Geometry: final body of the model. Coordinates: model frame, mm. A direction names the side the tool comes from. Give positions to 0.01 mm unless a question says otherwise; leave off trailing zeros. Order: outer loops, then holes, each group sorted by start corner. A loop starts at its lowest first (then second) coordinate and runs counter-clockwise, first axis right, second up. Notation, with made-up numbers: M 39,16.25 L 94,16.25 A20 cw 94,43.25 Z; hole C 70.25,-12.5 d4. An arc over 180 degrees is marked long. Write item = value, one per line. Start each with the question number.
from build123d import *

# Parameters (mm, degrees)
SKETCH_1_W            = 28
SKETCH_1_H            = 46
SKETCH_1_R            = 0.75
SKETCH_1_W_2          = 35.5
SKETCH_1_H_2          = 84
SKETCH_1_W_3          = 7
SKETCH_1_H_3          = 52
SKETCH_1_W_4          = 73
SKETCH_1_H_4          = 54
SKETCH_1_R_2          = 1
SKETCH_1_W_5          = 5
SKETCH_1_H_5          = 50
EXTRUDE_1_DEPTH       = 1
EXTRUDE_2_OUTLINE_W   = 73
EXTRUDE_2_OUTLINE_H   = 86
EXTRUDE_2_OUTLINE_W_2 = 71
EXTRUDE_2_OUTLINE_H_2 = 84
EXTRUDE_2_OUTLINE_W_3 = 1
EXTRUDE_2_OUTLINE_H_3 = 46
EXTRUDE_2_DEPTH       = 10
SKETCH_1_4_W          = 7
SKETCH_1_4_H          = 52
SKETCH_1_4_W_2        = 5
SKETCH_1_4_H_2        = 50
EXTRUDE_3_DEPTH       = 4
SKETCH_1_5_R          = 0.75
SKETCH_1_5_R_2        = 1
EXTRUDE_4_DEPTH       = 5
SKETCH_2_W            = 10
SKETCH_2_H            = 5
CUT_EXTRUDE_2_DEPTH   = 10


# Read off the part's stored shape, not the designer's step: the extrude step
with BuildPart() as part:
    # Sketch 1 → Extrude 1 (new body)
    # profile 1 of 10: a face of its own
    with BuildSketch(Plane(origin=(0, 0, 0), x_dir=(1, 0, 0), z_dir=(0, 1, 0))):
        with Locations((-15, 62)):
            Rectangle(SKETCH_1_W, SKETCH_1_H)
        with Locations(Location((-24, 43, 0), (0, 0, 270))):
            Circle(SKETCH_1_R, mode=Mode.SUBTRACT)
        with Locations(Location((-4, 43, 0), (0, 0, 270))):
            Circle(SKETCH_1_R, mode=Mode.SUBTRACT)
        with Locations(Location((-24, 81, 0), (0, 0, 270))):
            Circle(SKETCH_1_R, mode=Mode.SUBTRACT)
        with Locations(Location((-4, 81, 0), (0, 0, 270))):
            Circle(SKETCH_1_R, mode=Mode.SUBTRACT)
    # profile 2 of 10: a face of its own
    with BuildSketch(Plane(origin=(0, 0, 0), x_dir=(1, 0, 0), z_dir=(0, 1, 0))):
        with Locations((17.75, 42)):
            Rectangle(SKETCH_1_W_2, SKETCH_1_H_2)
        with Locations((5.5, 28.4)):
            Rectangle(SKETCH_1_W_3, SKETCH_1_H_3, mode=Mode.SUBTRACT)
    # profile 3 of 10: a face of its own
    with BuildSketch(Plane(origin=(0, 0, 0), x_dir=(1, 0, 0), z_dir=(0, 1, 0))):
        with Locations((53.25, 42)):
            Rectangle(SKETCH_1_W_2, SKETCH_1_H_2)
        with Locations((65.5, 28.4)):
            Rectangle(SKETCH_1_W_3, SKETCH_1_H_3, mode=Mode.SUBTRACT)
    # profile 4 of 10: a face of its own
    with BuildSketch(Plane(origin=(0, 0, 0), x_dir=(1, 0, 0), z_dir=(0, 1, 0))):
        with Locations((35.5, -28)):
            Rectangle(SKETCH_1_W_4, SKETCH_1_H_4)
        with Locations(Location((6.5, -43, 0), (0, 0, 270))):
            Circle(SKETCH_1_R_2, mode=Mode.SUBTRACT)
        with Locations(Location((64.5, -43, 0), (0, 0, 270))):
            Circle(SKETCH_1_R_2, mode=Mode.SUBTRACT)
        with Locations(Location((64.5, -16, 0), (0, 0, 270))):
            Circle(SKETCH_1_R_2, mode=Mode.SUBTRACT)
        with Locations(Location((6.5, -16, 0), (0, 0, 270))):
            Circle(SKETCH_1_R_2, mode=Mode.SUBTRACT)
    # profile 5 of 10: a face of its own
    with BuildSketch(Plane(origin=(0, 0, 0), x_dir=(1, 0, 0), z_dir=(0, 1, 0))):
        Polygon((72, 85), (35.5, 85), (35.5, 84), (71, 84), (71, 0), (35.5, 0), (35.5, -1), (72, -1), align=None)
    # profile 6 of 10: a face of its own
    with BuildSketch(Plane(origin=(0, 0, 0), x_dir=(1, 0, 0), z_dir=(0, 1, 0))):
        Polygon((35.5, 85), (-1, 85), (-1, 39), (-1, -1), (35.5, -1), (35.5, 0), (0, 0), (0, 84), (35.5, 84), align=None)
    # profile 7 of 10: a face of its own
    with BuildSketch(Plane(origin=(0, 0, 0), x_dir=(1, 0, 0), z_dir=(0, 1, 0))):
        with Locations((5.5, 28.4)):
            Rectangle(SKETCH_1_W_3, SKETCH_1_H_3)
        with Locations((5.5, 28.4)):
            Rectangle(SKETCH_1_W_5, SKETCH_1_H_5, mode=Mode.SUBTRACT)
    # profile 8 of 10: a face of its own
    with BuildSketch(Plane(origin=(0, 0, 0), x_dir=(1, 0, 0), z_dir=(0, 1, 0))):
        with Locations((5.5, 28.4)):
            Rectangle(SKETCH_1_W_5, SKETCH_1_H_5)
    # profile 9 of 10: a face of its own
    with BuildSketch(Plane(origin=(0, 0, 0), x_dir=(1, 0, 0), z_dir=(0, 1, 0))):
        with Locations((65.5, 28.4)):
            Rectangle(SKETCH_1_W_3, SKETCH_1_H_3)
        with Locations((65.5, 28.4)):
            Rectangle(SKETCH_1_W_5, SKETCH_1_H_5, mode=Mode.SUBTRACT)
    # profile 10 of 10: a face of its own
    with BuildSketch(Plane(origin=(0, 0, 0), x_dir=(1, 0, 0), z_dir=(0, 1, 0))):
        with Locations((65.5, 28.4)):
            Rectangle(SKETCH_1_W_5, SKETCH_1_H_5)
    extrude(amount=EXTRUDE_1_DEPTH)

    # Extrude 2 outline → Extrude 2 (add)
    # profile 1 of 2: a face of its own
    with BuildSketch(Plane(origin=(0, 0, 0), x_dir=(1, 0, 0), z_dir=(0, 1, 0))):
        with Locations((35.5, 42)):
            Rectangle(EXTRUDE_2_OUTLINE_W, EXTRUDE_2_OUTLINE_H)
        with Locations((35.5, 42)):
            Rectangle(EXTRUDE_2_OUTLINE_W_2, EXTRUDE_2_OUTLINE_H_2, mode=Mode.SUBTRACT)
    # profile 2 of 2: a face of its own
    with BuildSketch(Plane(origin=(0, 0, 0), x_dir=(1, 0, 0), z_dir=(0, 1, 0))):
        with Locations((-29.5, 62)):
            Rectangle(EXTRUDE_2_OUTLINE_W_3, EXTRUDE_2_OUTLINE_H_3)
    extrude(amount=EXTRUDE_2_DEPTH)

    # Sketch 1_4 → Extrude 3 (add)
    # profile 1 of 2: a face of its own
    with BuildSketch(Plane(origin=(0, 0, 0), x_dir=(1, 0, 0), z_dir=(0, 1, 0))):
        with Locations((5.5, 28.4)):
            Rectangle(SKETCH_1_4_W, SKETCH_1_4_H)
        with Locations((5.5, 28.4)):
            Rectangle(SKETCH_1_4_W_2, SKETCH_1_4_H_2, mode=Mode.SUBTRACT)
    # profile 2 of 2: a face of its own
    with BuildSketch(Plane(origin=(0, 0, 0), x_dir=(1, 0, 0), z_dir=(0, 1, 0))):
        with Locations((65.5, 28.4)):
            Rectangle(SKETCH_1_4_W, SKETCH_1_4_H)
        with Locations((65.5, 28.4)):
            Rectangle(SKETCH_1_4_W_2, SKETCH_1_4_H_2, mode=Mode.SUBTRACT)
    extrude(amount=EXTRUDE_3_DEPTH)

    # Sketch 1_5 → Extrude 4 (add)
    with BuildSketch(Plane(origin=(0, 0, 0), x_dir=(1, 0, 0), z_dir=(0, 1, 0))):
        with Locations(Location((-4, 43, 0), (0, 0, 270))):
            Circle(SKETCH_1_5_R)
        with Locations(Location((-24, 43, 0), (0, 0, 270))):
            Circle(SKETCH_1_5_R)
        with Locations(Location((-24, 81, 0), (0, 0, 270))):
            Circle(SKETCH_1_5_R)
        with Locations(Location((-4, 81, 0), (0, 0, 270))):
            Circle(SKETCH_1_5_R)
        with Locations(Location((6.5, -16, 0), (0, 0, 270))):
            Circle(SKETCH_1_5_R_2)
        with Locations(Location((64.5, -16, 0), (0, 0, 270))):
            Circle(SKETCH_1_5_R_2)
        with Locations(Location((64.5, -43, 0), (0, 0, 270))):
            Circle(SKETCH_1_5_R_2)
        with Locations(Location((6.5, -43, 0), (0, 0, 270))):
            Circle(SKETCH_1_5_R_2)
    extrude(amount=EXTRUDE_4_DEPTH)

    # Sketch 2 → Cut-Extrude 2 (cut)
    with BuildSketch(Plane.XY.offset(-84)):
        with Locations((48, 7.5)):
            Rectangle(SKETCH_2_W, SKETCH_2_H)
    extrude(amount=-CUT_EXTRUDE_2_DEPTH, mode=Mode.SUBTRACT)


solid = part.part
1) Draft query along X for faces 4 (the flat face through (35, 5, 1)), 5 (the flat face through (69, 2, -28)). Return one class per face: pulls with the +X half, pulls with the -X half, needs draft (parallel to the pull), parting line crosses it, or undercut.
2) Cut plane C-C (z = 3). Return loops of the section in (x, y).
3) Cut plane A-A (z = -75). Return loops of the section in (x, y), plus the area to 3 significant figures.
4) Cut plane B-B (x = 36). Return loops of the section in (y, z), plus the area to 3 significant figures.
5) Cut plane D-D (x = -21.5). Return loops of the section in (y, z).
6) Access query for faces 1 (the flat face through (-19.9, 0.5, -39)), 2 (the flat face through (2, 2, -28)), 3 (the flat face through (-29, 5, -62)). Directions: +Z, -Z, +X, -X, +Y, -Y. A direction counts if a zero-diameter tool reaches every point of the face in a straight line with its end or side. Return the directions, or none.
7) Ray query, L1, parallel to X at y = 4.75, z = -42; L2, parallel to X at y = 3.25, z = -38; L3, parallel to Z at x = 9, y = 5.75. Return the intervals inside material, ascending.
8) Pin query (flat end, axial travel): pin 1 Ø5 at (y, z) = (6.5, -25) entering from -X; pin 2 Ø1.5 at (x, y) = (8.5, 6) entering from +Z; pin 3 Ø1.5 at (x, y) = (5, 2) entering from +Z. Return the tip coordinate at first contact, or that it passes through.
Reply:
q1.face_4 = needs draft
q1.face_5 = undercut
q2.outline = M -1,0 L 72,0 L 72,1 L -1,1 Z
q3.outline = M -30,0 L 72,0 L 72,10 L 71,10 L 71,1 L 0,1 L 0,10 L -1,10 L -1,1 L -29,1 L -29,10 L -30,10 Z
q3.area = 129 mm²
q4.outline = M 0,-85 L 10,-85 L 10,-84 L 1,-84 L 1,0 L 10,0 L 10,1 L 1,1 L 1,55 L 0,55 Z
q4.area = 158 mm²
q5.outline = M 0,-85 L 1,-85 L 1,-39 L 0,-39 Z
q6.face_1 = +Z, -X, +Y, -Y
q6.face_2 = +Y
q6.face_3 = +Z, -Z, +Y
q7.L1 = -30 to -29, -1 to 0, 71 to 72
q7.L2 = -1 to 0, 2 to 3, 8 to 9, 62 to 63, 68 to 69, 71 to 72
q7.L3 = -85 to -84, 0 to 1
q8.pin_1 = -1
q8.pin_2 = 1
q8.pin_3 = 43.66
